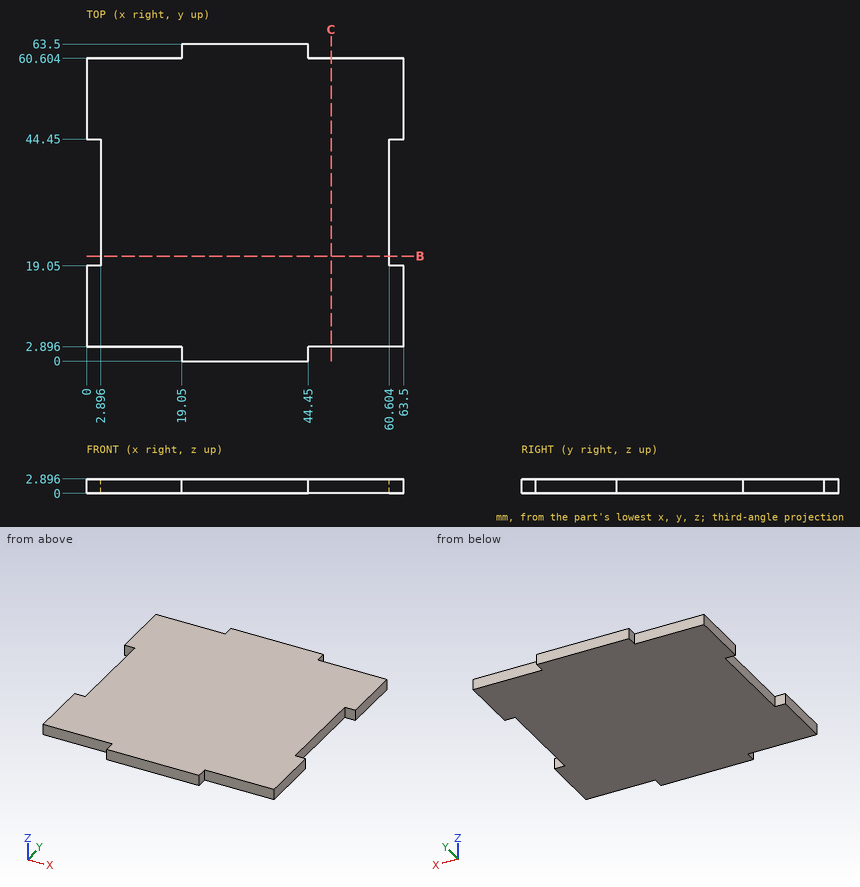
Check sheet for the drawn part. Datum: minimum x, y, z corner. Units: mm. Round coordinates to 2 decimals unless told otherwise and drop trailing zeros. Order: outer loops, then holes, each group sorted by start corner. A loop starts at its lowest first (then second) coordinate and runs counter-clockwise, first axis right, second up.
(1) Scan line: probe 1 along X at (y, z) = (33, 0.9) (1 decimal). Record every from-to range of solid material in increasing order.
(2) Go/stop test with flat-tipped pins: P1, Ø0.9, axis at x = 62, z = 1.5, coming from the -Y side; P2, Ø1.4, axis at x = 62, z = 2, coming from the +Y side; P3, Ø1.4, axis at y = 1, z = 2, coming from the +X side. Record where each tip stops, or that it passes through.
(3) Cross-section at B-B, the plane y = 21. Enter the section's corners in (x, z) (1 decimal), and give its area (3 significant figures).
Check sheet entries:
1. probe 1: x = 2.9 to 60.6
2. P1: stops at y = 2.9
2. P2: stops at y = 60.6
2. P3: stops at x = 44.45
3. outline: (2.9, 0) - (60.6, 0) - (60.6, 2.9) - (2.9, 2.9) - close
3. area: 167 mm2
